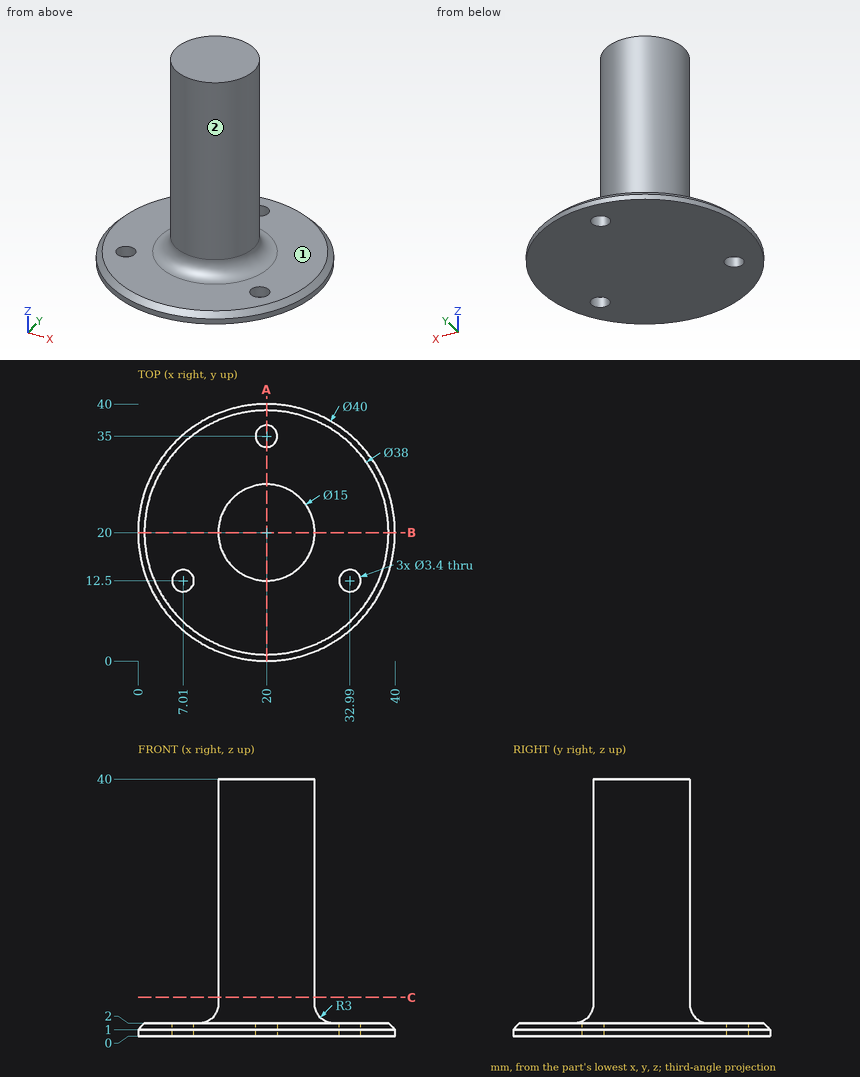
Study the drawing (mm; zero at the part's minimum x, y, z) and answer. Give positions to 0.01 mm unless a question says otherwise; leave off trailing zeros. Write each loop counter-clockwise with the first axis right and the second up, starting at its lowest first coordinate (ties: lowest second). Pieces come first, ordered by that corner, then holes. Notation, with made-up numbers: M -40,13 L -9,13 A10 cw -9,21 Z; hole C 8,40.25 d3. An arc over 180 degrees is marked long. Put each result on its own line as item: value. Start each with the question number.
1. The part is cut by section B-B, the plane y = 20. Give the vertices of the cut face in (x, z), and give its area (3 significant figures).
2. Each of these flat-tipped pins is pushed along its axis until it touches: pin 1 Ø12 at (x, z) = (13, 17.5) entering from -Y; pin 2 Ø2 at (x, y) = (7.01, 12.5) entering from +Z; pin 3 Ø10 at (y, z) = (16, 24.5) entering from +X; pin 4 Ø8 at (y, z) = (26.5, 7.5) entering from -X. Where does it stop, or does it pass through?
3. The part is cut by section C-C, the plane z = 6. Give the vertices of the cut face in (x, y), and give its area (3 significant figures).
4. Consider line 1 along Y through (x, z) = (20, 0.5); line 2 along X through (y, z) = (12, 1) (1 decimal); line 3 along Z through (x, y) = (23.5, 36.5). Determine where each line is inside the solid, lowest interval first.
5. The part is cut by section A-A, the plane x = 20. Give the vertices of the cut face in (y, z), and give its area (3 significant figures).
6. For a pull along X with two mould halves and no side action, classify the marked faces 1 and 2 as released by +X, released by -X, zero draft, split by the parting line, or undercut.
Final values:
1. outline: M 0,0 L 40,0 L 40,1 L 39,2 L 30.5,2 A3 cw 27.5,5 L 27.5,40 L 12.5,40 L 12.5,5 A3 cw 9.5,2 L 1,2 L 0,1 Z
1. area: 653 mm²
2. pin 1: stops at y = 12.57
2. pin 2: passes through
2. pin 3: stops at x = 27.5
2. pin 4: stops at x = 12.93
3. outline: C 20,20 d15
3. area: 177 mm²
4. line 1: y = 0 to 33.3, 36.7 to 40
4. line 2: x = 1.7 to 5.4, 8.6 to 31.4, 34.6 to 38.3
4. line 3: z = 0 to 2
5. outline: M 0,0 L 33.3,0 L 33.3,2 L 30.5,2 A3 cw 27.5,5 L 27.5,40 L 12.5,40 L 12.5,5 A3 cw 9.5,2 L 1,2 L 0,1 Z; M 36.7,0 L 40,0 L 40,1 L 39,2 L 36.7,2 Z
5. area: 646 mm²
6. face 1: zero draft
6. face 2: split by the parting line
